```python
from build123d import *

# Parameters (mm, degrees)
F0_W     = 127
F0_H     = 50.8
F1_DEPTH = 19.05
F2_W     = 88.9
F2_H     = 13.97
F3_DEPTH = 38.1
F4_R     = 5.08
F5_R     = 12.7


with BuildPart() as f1:
    # F0 (on Top) → F1 (new body)
    with BuildSketch(Plane.XY):
        Rectangle(F0_W, F0_H)
    extrude(amount=F1_DEPTH)

    # F2 (on face) → F3 (cut)
    with BuildSketch(Plane.XZ.offset(25.4)):
        with Locations((0, 6.985)):
            Rectangle(F2_W, F2_H)
    extrude(amount=-F3_DEPTH, mode=Mode.SUBTRACT)

    # F4
    f4_edges = [f1.edges().sort_by_distance(p)[0] for p in [
        (44.45, -6.35, 13.97),
        (0, 12.7, 13.97),
        (-44.45, -6.35, 13.97),
    ]]
    fillet(f4_edges, radius=F4_R)

    # F5
    f5_edges = [f1.edges().sort_by_distance(p)[0] for p in [
        (-63.5, 25.4, 9.525),
        (63.5, 25.4, 9.525),
        (-63.5, -25.4, 9.525),
        (63.5, -25.4, 9.525),
    ]]
    fillet(f5_edges, radius=F5_R)


solid = f1.part
```
Geometry check sheet. Reference: the model listing, model coordinates, mm. A direction names the side the tool comes from. Give positions to 0.01 mm unless a question says otherwise; leave off trailing zeros. Order: outer loops, then holes, each group sorted by start corner. A loop starts at its lowest first (then second) coordinate and runs counter-clockwise, first axis right, second up.
1. Access from +Z, -Z, +X, -X, +Y, -Y to the whole of each face (thin tool, end or side, straight path). Record for faces 5 (the face through (-44.45, -7, 4)), 6 (the face through (59.88, 21.58, 9.66)).
2. Section check D-D, the plane y = 3. Enter the section's corners in (x, z), and give its area (3 significant figures).
3. Section check B-B, the plane x = -35. Enter the section's corners in (y, z).
4. Thickness scan on L1, parallel to X at y = 7.5, z = 9; L2, parallel to Y at x = -22, z = 2; L3, parallel to Y at x = -51.5, z = 4. Record the ranges inside material, lowest first.
5. Section check C-C, the plane z = 3. Enter the section's corners in (x, y).
6. Release check for a two-part mould opening along X. For faces 1 (the face through (-1, 12.7, 5)), 2 (the face through (0.622, 11.172, 12.521)), 3 (the face through (59.68, -21.78, 9.66)), 4 (the face through (-59.68, -21.78, 9.66)) record: pulls with the +X half, pulls with the -X half, needs draft (parallel to the pull), parting line crosses it, or undercut.
7. Section check A-A, the plane y = -15. Enter the section's corners in (x, z).
8. Gauge pin test, flat ends, axial feed: pin 1 Ø2.5 at (x, z) = (20.5, 2.5) entering from -Y; pin 2 Ø10 at (y, z) = (13.5, 15.5) entering from +X; pin 3 Ø10 at (x, y) = (17, -12) entering from -Z. Record the tip position at first contact, or that the pin passes through.
Values follow:
1. face 5: -Z, -Y
1. face 6: +Z, -Z, +X, +Y
2. outline: (-63.5, 0) - (-44.45, 0) - (-44.45, 8.89) arc R5.08 cw to (-39.37, 13.97) - (39.37, 13.97) arc R5.08 cw to (44.45, 8.89) - (44.45, 0) - (63.5, 0) - (63.5, 19.05) - (-63.5, 19.05) - close
2. area: 1,190 mm2
3. outline: (-25.4, 13.97) - (7.62, 13.97) arc R5.08 cw to (12.7, 8.89) - (12.7, 0) - (25.4, 0) - (25.4, 19.05) - (-25.4, 19.05) - close
4. L1: x = -63.5 to -44.45, 44.45 to 63.5
4. L2: y = 12.7 to 25.4
4. L3: y = -25.38 to 25.38
5. outline: (-63.5, -12.7) arc R12.7 ccw to (-50.8, -25.4) - (-44.45, -25.4) - (-44.45, 12.7) - (44.45, 12.7) - (44.45, -25.4) - (50.8, -25.4) arc R12.7 ccw to (63.5, -12.7) - (63.5, 12.7) arc R12.7 ccw to (50.8, 25.4) - (-50.8, 25.4) arc R12.7 ccw to (-63.5, 12.7) - close
6. face 1: undercut
6. face 2: undercut
6. face 3: pulls with the +X half
6. face 4: pulls with the -X half
7. outline: (-63.29, 0) - (-44.45, 0) - (-44.45, 8.89) arc R5.08 cw to (-39.37, 13.97) - (39.37, 13.97) arc R5.08 cw to (44.45, 8.89) - (44.45, 0) - (63.29, 0) - (63.29, 19.05) - (-63.29, 19.05) - close
8. pin 1: stops at y = 12.7
8. pin 2: stops at x = 63.5
8. pin 3: stops at z = 13.97
